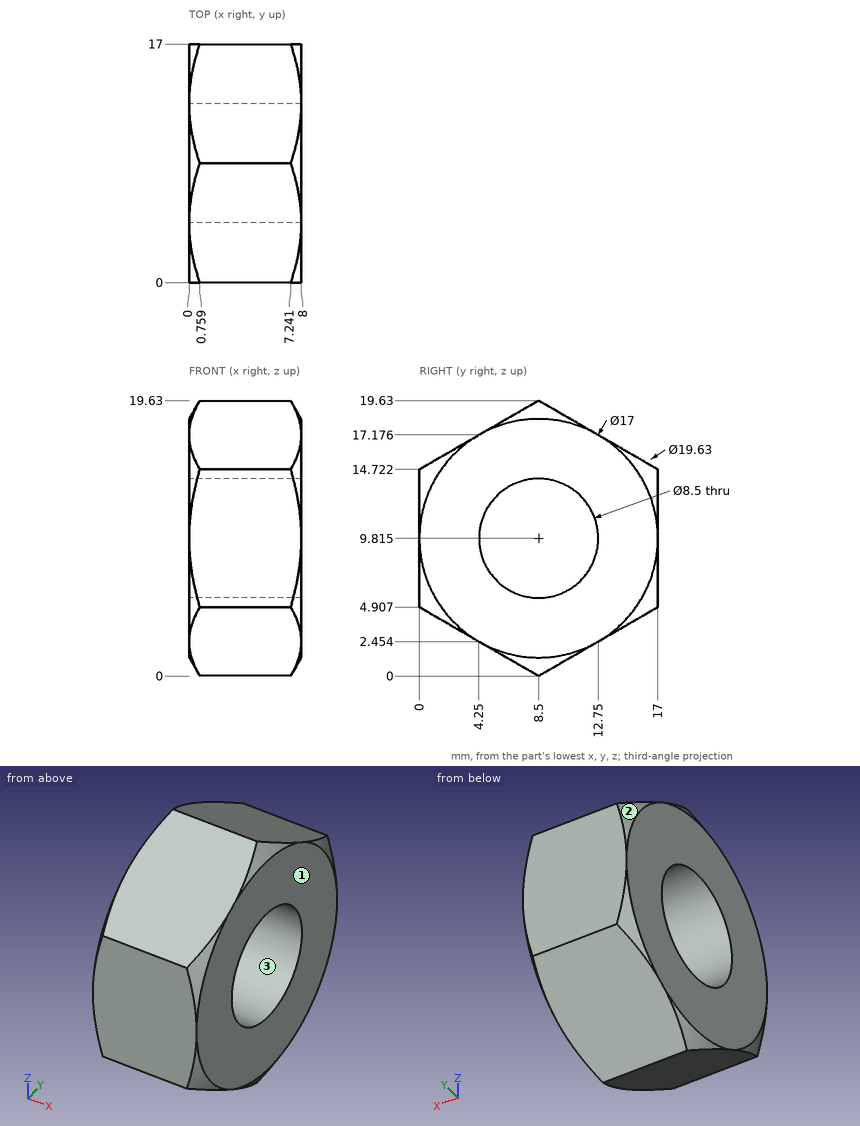
Part print with two shaded views. Sizes in mm from the minimum x, y, z corner. Give positions to 0.01 mm unless a question says otherwise; leave off trailing zeros. One line per question, with ' | ' between items.
Q1. Pull direction Y, two halves, no side cores. Call the marked faces 1, 2 and 3: pulls with the +Y half, pulls with the -Y half, needs draft (parallel to the pull), parting line crosses it, or undercut.
Filled sheet:
face 1: needs draft | face 2: pulls with the +Y half | face 3: undercut
Q2. Drill centre lines: line 1 along Z through (x, y) = (0.75, 11.5) (1 decimal); line 2 along Y through (x, z) = (1.75, 9); line 3 along Y through (x, z) = (6, 8). Where is each one in solid material? Low to high. Write a range as [from, to].
Filled sheet:
line 1: z = [1.7, 6.8], [12.8, 17.9] | line 2: y = [0, 4.33], [12.67, 17] | line 3: y = [0, 4.66], [12.34, 17]
Q3. Drop flat-ended pins along their axis: pin 1 (2 mm diameter, centred on x = 2, y = 12, fed in from -Z); pin 2 (1 mm diameter, centred on x = 7, z = 17.5, fed in from +Y) (1 decimal); pin 3 (1.5 mm diameter, centred on y = 9, z = 7, fed in from -X). Give the stop position or say it passes through.
Filled sheet:
pin 1: stops at z = 1.44 | pin 2: stops at y = 13.1 | pin 3: passes through
